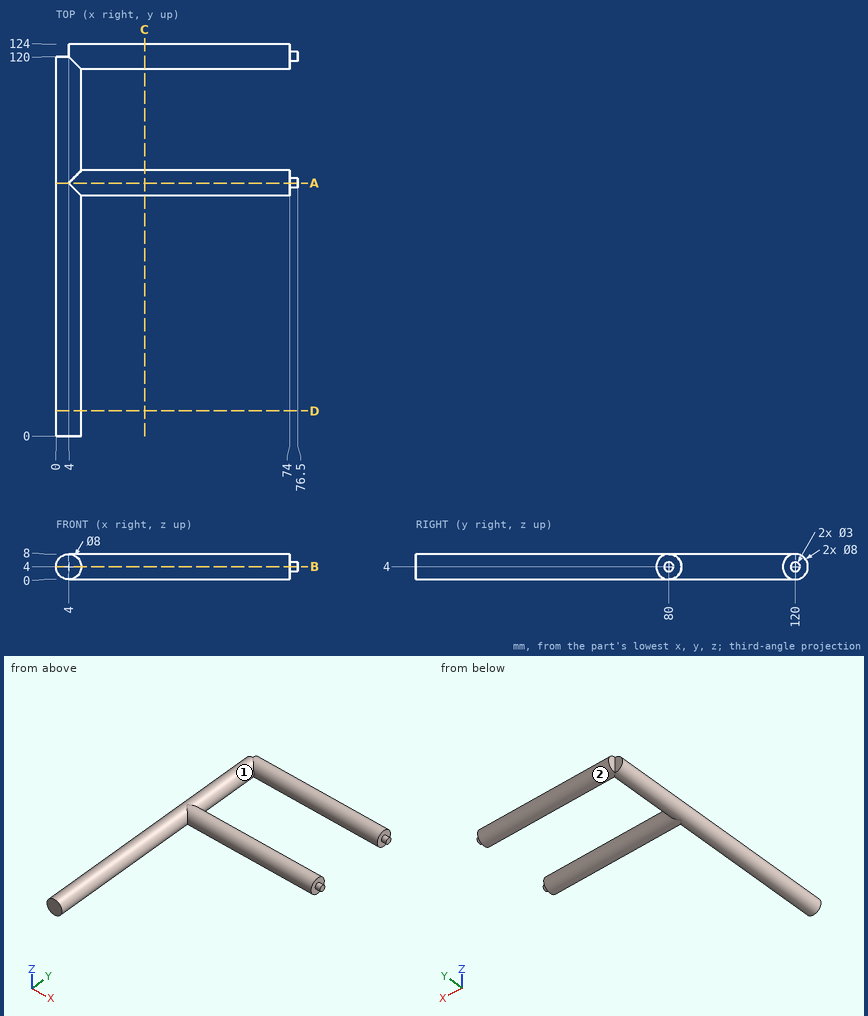
Source: three-view drawing plus pictorial views. Frame: mm from the lowest corner of the part. A direction names the side the tool comes from. Give positions to 0.01 mm unless a question says otherwise; leave off trailing zeros. Order: outer loops, then holes, each group sorted by start corner. A loop starts at its lowest first (then second) coordinate and runs counter-clockwise, first axis right, second up. Notation, with made-up numbers: (81, -9) - (115, -9) arc R31 ccw to (115, 26) - close; hole circle Ø6 at (7.5, 34.5). An arc over 180 degrees is marked (long way). Put each result on its own line as item: value.
Item 1: Section query C-C, the plane x = 28. Return loops of the section in (y, z).
Found:
outline: circle Ø8 at (80, 4); circle Ø8 at (120, 4)
Item 2: Ray query, L1, parallel to X at y = 67, z = 3.75; L2, parallel to Y at x = 12, z = 2.25; L3, parallel to Y at x = 10.5, z = 6.5. Return the intervals inside material, ascending. Write a range as from..to.
Found:
L1: x = 0.01..7.99
L2: y = 76.4..83.6, 116.4..123.6
L3: y = 76.88..83.12, 116.88..123.12
Item 3: Section query B-B, the plane z = 4. Return loops of the section in (x, y).
Found:
outline: (0, 0) - (8, 0) - (8, 76) - (74, 76) - (74, 78.5) - (76.5, 78.5) - (76.5, 81.5) - (74, 81.5) - (74, 84) - (8, 84) - (8, 116) - (74, 116) - (74, 118.5) - (76.5, 118.5) - (76.5, 121.5) - (74, 121.5) - (74, 124) - (4, 124) - (4, 120) - (0, 120) - close
Item 4: Contact query for flat-ended pins moving along their axis: pin 1 (3 mm diameter, centred on x = 52, z = 1.5, fed in from +Y); pin 2 (3 mm diameter, centred on y = 85.5, z = 6, fed in from -X); pin 3 (4 mm diameter, centred on x = 25, z = 4, fed in from -Y). Output: stop coordinate, or through.
Found:
pin 1: stops at y = 123.87
pin 2: stops at x = 0.03
pin 3: stops at y = 76
Item 5: Section query A-A, the plane y = 80. Return loops of the section in (x, z), then the cut area to 3 significant figures.
Found:
outline: (4, 0) - (74, 0) - (74, 2.5) - (76.5, 2.5) - (76.5, 5.5) - (74, 5.5) - (74, 8) - (4, 8) arc R4 ccw to start
area: 593 mm^2
Item 6: Section query D-D, the plane y = 8. Return loops of the section in (x, z), then the cut area to 3 significant figures.
Found:
outline: circle Ø8 at (4, 4)
area: 50.3 mm^2
Item 7: Access query for the marked faces 1 and 2. Directions: +Z, -Z, +X, -X, +Y, -Y. A direction counts if a zero-diameter tool reaches every point of the face in a straight line with its end or side. Return the directions, or none.
Found:
face 1: none
face 2: +X
